Source: CAD feature listing. Evaluate the final solid. Frame: model axes, mm. A direction names the side the tool comes from. Give positions to 0.01 mm unless a question says otherwise; leave off trailing zeros. Order: outer loops, then holes, each group sorted by start corner. A loop starts at its lowest first (then second) coordinate and runs counter-clockwise, first axis right, second up. Notation, with made-up numbers: M -34.5,-12.75 L -7.5,-12.75 A17 ccw -7.5,-1.75 Z; hole C -23.5,1 d3. An arc over 180 degrees is marked long. Answer as a JSON object with one key per item and string values. Group by question number.
1. Section query C-C (y = 8.5). Output: boundary loops of the cut face in (x, z).
2. Section query B-B (x = -0.75). Output: boundary loops of the cut face in (y, z).
3. Section query D-D (x = 11.5). Output: boundary loops of the cut face in (y, z), plus the area to 3 significant figures.
4. Pull-direction query (Y, two-part tool) for faces 1 (the cylindrical face through (7.526, 11.805, 3.916)), 2 (the cylindrical face through (4.3, -12.4, 1)), 3 (the flat face through (0, -3, 0)); classes: +Y half, -Y half, draft (parallel to the pull), parting line (faces both ways), or undercut.
5. Pin query (flat end, axial travel): P1, Ø5, axis at x = 10.5, z = 2, coming from the +Y side; P2, Ø5, axis at y = 4.5, z = 6.5, coming from the +X side; P3, Ø0.6, axis at x = 12, y = 0, coming from the +Z side; P4, Ø12.5, axis at x = 5.5, y = -3, coming from the +Z side. Return the tip coordinate at first contact, or that it passes through.
6. Section query A-A (z = 7). Output: boundary loops of the cut face in (x, y), plus the area to 3 significant figures.
7. Material intervals for L1, parallel to Y at x = 0, z = -0.55; L2, parallel to Y at x = -11.5, z = 4; L3, parallel to Z at x = 4, y = -9.25, sorted ascending. Write a range as [from, to].
8. Set-up query: faces 4 (the flat face through (6, -12, 7)), 5 (the cylindrical face through (10.5, 0, 6.1)), 6 (the cylindrical face through (0, 13, 5)). Return all of +Z, -Z, +X, -X, +Y, -Y with unobstructed straight access to the full face (end or side cutting, diameter ignored); none if empty.
from build123d import *

# Parameters (mm, degrees)
SKETCH_R        = 14
PAD_DEPTH       = 12
SKETCH001_R     = 12.5
POCKET_DEPTH    = 10
SKETCH002_R     = 1.25
SKETCH002_R_2   = 2
POCKET001_DEPTH = 5
SKETCH003_R     = 2
PAD001_DEPTH    = 10
SKETCH004_R     = 1
POCKET002_DEPTH = 8
SKETCH005_R     = 6.725
POCKET003_DEPTH = 20
SKETCH006_W     = 12
SKETCH006_H     = 6
POCKET004_DEPTH = 20
POCKET005_DEPTH = 20
FILLET_R        = 1


with BuildPart() as part:
    # Sketch → Pad (new body)
    with BuildSketch(Plane.XY.offset(4)):
        Circle(SKETCH_R)
    extrude(amount=PAD_DEPTH)

    # Sketch001 (on Face3 of Pad) → Pocket (cut)
    with BuildSketch(Plane.XY.offset(16)):
        Circle(SKETCH001_R)
    extrude(amount=-POCKET_DEPTH, mode=Mode.SUBTRACT)

    # Sketch002 (on Face5 of Pocket) → Pocket001 (cut)
    with BuildSketch(Plane.XY.offset(6)):
        Circle(SKETCH002_R)
        with Locations((0, 7)):
            Circle(SKETCH002_R_2)
    extrude(amount=-POCKET001_DEPTH, mode=Mode.SUBTRACT)

    # Sketch003 (on Face7 of Pocket001) → Pad001 (join)
    with BuildSketch(Plane.XY.offset(6)):
        with Locations((-11.5, 0)):
            Circle(SKETCH003_R)
        with Locations((11.5, 0)):
            Circle(SKETCH003_R)
    extrude(amount=PAD001_DEPTH)

    # Sketch004 (on Face3 of Pad001) → Pocket002 (cut)
    with BuildSketch(Plane.XY.offset(16)):
        with Locations((-11.5, 0)):
            Circle(SKETCH004_R)
        with Locations((11.5, 0)):
            Circle(SKETCH004_R)
    extrude(amount=-POCKET002_DEPTH, mode=Mode.SUBTRACT)

    # Sketch005 → Pocket003 (cut)
    with BuildSketch(Plane.XZ):
        with Locations((0, 17.725)):
            Circle(SKETCH005_R)
    extrude(amount=-POCKET003_DEPTH, mode=Mode.SUBTRACT)

    # Sketch006 → Pocket004 (cut)
    with BuildSketch(Plane.XZ):
        with Locations((0, 13)):
            Rectangle(SKETCH006_W, SKETCH006_H)
    extrude(amount=POCKET004_DEPTH, mode=Mode.SUBTRACT)

    # Sketch007 → Pocket005 (cut)
    with BuildSketch(Plane.XZ):
        with BuildLine():
            ThreePointArc((5.3, 8.881966), (4.3, 11.5), (3.3, 8.881966))
            Line((3.3, 8.881966), (3.3, 8))
            ThreePointArc((3.3, 8), (4.3, 7), (5.3, 8))
            Line((5.3, 8), (5.3, 8.881966))
        make_face()
    pocket005 = extrude(amount=POCKET005_DEPTH, mode=Mode.SUBTRACT)

    # Mirrored: Pocket005 across Sketch007 V_Axis
    add(pocket005.mirror(Plane(origin=(0, 0, 0), x_dir=(0, -1, 0), z_dir=(1, 0, 0))), mode=Mode.SUBTRACT)

    # Fillet
    fillet_edges = [part.edges().sort_by_distance(p)[0] for p in [
        (3.3, -12.831024, 8.881966),
        (5.3, -12.139393, 8.881966),
        (-3.3, -12.831024, 8.881966),
        (-5.3, -12.139393, 8.881966),
        (-2.8, -12.949753, 10),
        (2.8, -12.949753, 10),
    ]]
    fillet(fillet_edges, radius=FILLET_R)


with BuildPart() as part_1:
    # Body placement: moved
    add(part.part.moved(Location((0, 0, -6))))


solid = part_1.part
Answer sheet:
{
 "1": {"outline": "M -11.12,-2 L -1.32,-2 L -1.32,0 L -9.17,0 L -9.17,10 L -11.12,10 Z; M 1.32,-2 L 11.12,-2 L 11.12,10 L 9.17,10 L 9.17,0 L 1.32,0 Z"},
 "2": {"outline": "M -13.98,-2 L -1,-2 L -1,0 L -12.48,0 L -12.48,4 L -13.98,4 Z; M 1,-2 L 5.15,-2 L 5.15,0 L 1,0 Z; M 8.85,-2 L 13.98,-2 L 13.98,5.04 L 12.48,5.04 L 12.48,0 L 8.85,0 Z"},
 "3": {"outline": "M -7.98,-2 L 7.98,-2 L 7.98,10 L 4.9,10 L 4.9,0 L 2,0 L 2,10 L 1,10 L 1,2 L -1,2 L -1,10 L -2,10 L -2,0 L -4.9,0 L -4.9,10 L -7.98,10 Z", "area": "118 mm^2"},
 "4": {"face 1": "parting line", "face 2": "draft", "face 3": "undercut"},
 "5": {"P1": "y = 11.49", "P2": "x = 13.86", "P3": "z = 2", "P4": "z = 10"},
 "6": {"outline": "M -12.37,-1.8 A2 ccw long -12.37,1.8 A12.5 cw -4.79,11.55 L -4.79,13.16 A14 ccw -6,-12.65 L -6,-10.97 A12.5 cw Z; M 4.79,11.55 A12.5 cw 12.37,1.8 A2 ccw long 12.37,-1.8 A12.5 cw 6,-10.97 L 6,-12.65 A14 ccw 4.79,13.16 Z; hole C -11.5,0 d2; hole C 11.5,0 d2", "area": "105 mm^2"},
 "7": {"L1": "[-14, -1.25], [1.25, 5], [9, 14]", "L2": "[-7.98, -4.9], [-2, -1], [1, 2], [4.9, 7.98]", "L3": "[-2, 0]"},
 "8": {"face 4": "+Z, -Y", "face 5": "+Z", "face 6": "+Z, +Y"}
}
